CAD build for the part. Positions are in the model's coordinates, mm. Coordinates: 2 decimals unless noted, no trailing zeros. Loops run counter-clockwise (first coordinate to the right, second up) from the corner with the lowest first, then second, coordinate; pieces in that order, holes last. Notation, with made-up numbers: (16.5, 28.5) -> (54.5, 28.5) arc R14 ccw to (54.5, 39.5) -> close; hole circle Ø11 at (24, 2.25). An arc over 180 degrees is marked (long way). Write each question's results on one line, items separated by ' | '.
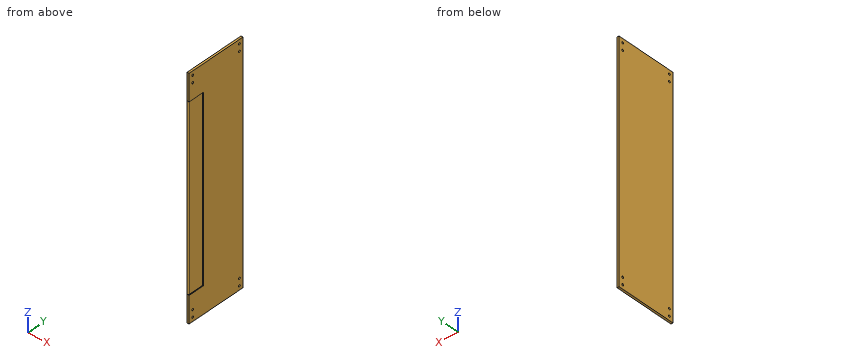
Autodesk Inventor part; units mm, degrees
ref_plane "YZ Plane" through (0, 0, 0) normal (1, 0, 0) x (0, 1, 0)
ref_plane "XZ Plane" through (0, 0, 0) normal (0, 1, 0) x (-1, 0, 0)
ref_plane "XY Plane" through (0, 0, 0) normal (0, 0, 1) x (1, 0, 0)
sketch "Sketch1" plane through (0, 0, 0) normal (1, 0, 0) x (0, 1, 0)
  line L0 (75, 285) -> (-75, 285)
  line L1 (-75, 285) -> (-75, -285)
  line L2 (-75, -285) -> (75, -285)
  line L3 (75, -285) -> (75, 285)
  line L4 (75, 285) -> (-75, -285) construction
  line L5 (-75, 285) -> (75, -285) construction
  point P0 (0, 0)
  dimension "d0" = 150
  dimension "d1" = 570
extrude "Plate1" add sketch "Sketch1" along normal blind 5
sketch "Sketch2" plane through (5, 0, 0) normal (1, 0, 0) x (0, 0, -1)
  line L0 (-285, 75) -> (-285, -75)
  line L1 (-285, -75) -> (-285, -35)
  line L2 (-285, -75) -> (285, -75)
  line L3 (0, -75) -> (-220, -75)
  line L4 (0, -75) -> (220, -75)
  line L5 (220, -75) -> (220, -35)
  line L6 (220, -35) -> (0, -35)
  line L7 (0, -35) -> (0, -75)
  line L8 (0, -75) -> (-220, -75)
  line L9 (-220, -75) -> (-220, -35)
  line L10 (-220, -35) -> (0, -35)
  line L11 (0, -35) -> (0, -75)
  point P0 (0, 0)
  dimension "d3" = 40
  dimension "d4" = 220
  dimension "d5" = 220
  dimension "d6" = 40
  dimension "d7" = 220
  dimension "d8" = 40
extrude "Cut1" cut sketch "Sketch2" against normal blind 5
sketch "Sketch3" plane through (5, -35, -220) normal (0, -1, 0) x (1, 0, 0)
  line L0 (0, 440) -> (0, 0)
  line L1 (0, 440) -> (-5, 440)
  line L2 (-5, 0) -> (-5, 440)
  line L3 (0, 0) -> (-5, 0)
  line L4 (-5, 0) -> (-5, 440)
  line L5 (-5, 440) -> (-2, 440)
  line L6 (-2, 440) -> (-2, 0)
  line L7 (-2, 0) -> (-5, 0)
  line L8 (-5, 0) -> (-5, 440)
  point P0 (-5, 220)
  dimension "d11" = 3
  dimension "d12" = 440
extrude "Extrusion1" add sketch "Sketch3" along normal blind 40 contours L6 L3 L2 L1
fillet "Fillet1" radius 3 1 edges at (3, -75, 0)
sketch "Sketch4" plane through (5, 0, 0) normal (1, 0, 0) x (0, 0, -1)
  line L0 (-285, -75) -> (-285, 75)
  line L1 (-220, -75) -> (-285, -75)
  circle A0 centre (-275, -65) radius 2.5
  circle A1 centre (-258, -65) radius 2.5
  line L2 (-285, 0) -> (-275, 0)
  circle A2 centre (-275, 65) radius 2.5
  circle A3 centre (-258, 65) radius 2.5
  point P0 (0, 0)
  dimension "d16" = 10
  dimension "d17" = 10
  dimension "d18" = 5
  dimension "d19" = 17
  dimension "d20" = 5
extrude "Extrusion2" cut sketch "Sketch4" against normal mid plane 40
mirror "Mirror1" about plane through (0, 0, 0) normal (0, 0, 1) of "Extrusion2"
equation "\"d9\" = Thickness"
equation "\"d2\" = Thickness"
equation "\"BendRadius\" = Thickness"
equation "\"BendReliefWidth\" = Thickness"
equation "\"BendReliefDepth\" = 0.5 * Thickness"
equation "\"TransitionRadius\" = BendRadius"
equation "\"JacobiRadiusSize\" = BendRadius"
equation "\"GapSize\" = Thickness"
properties part number "elevatotr"
1) Slice it at B-B (y = -40). Write the cut outline in (x, z).
Outcome:
outline: (0, -285) -> (5, -285) -> (5, -220) -> (3, -220) -> (3, 220) -> (5, 220) -> (5, 285) -> (0, 285) -> close
2) Slice it at A-A (x = 4.15). Count the separate pieces of the cut face and the enclosed holes in it, then the cut area to 3 significant figures.
Outcome:
separate pieces: 1 | enclosed holes: 8 | area: 67,700 mm^2
3) Drill centre lines: L1, parallel to Y at x = 1.5, z = -258; L2, parallel to Y at x = 4.6, z = -110; L3, parallel to X at y = -39.5, z = 56.5. Where is each one in solid material? Low to high. Write a range as from..to.
Outcome:
L1: y = -75..-67.5, -62.5..62.5, 67.5..75 | L2: y = -35..75 | L3: x = 0..3
4) Pin check, flat tip, straight feed: pin 1 (4.5 mm diameter, centred on y = -65, z = 275, fed in from -X). Stop position of the tip, or through.
Outcome:
pin 1: passes through
